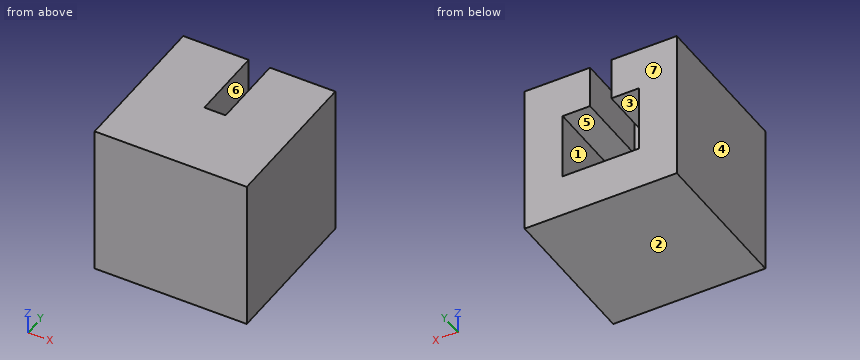
```python
from build123d import *

# Parameters (mm, degrees)
SKETCH1_W           = 12.7
SKETCH1_H           = 12.7
BOSS_EXTRUDE1_DEPTH = 12.7
SKETCH2_W           = 1.778
SKETCH2_H           = 3.560002412
CUT_EXTRUDE1_DEPTH  = 6.35


with BuildPart() as part:
    # Sketch1 → Boss-Extrude1 (new body)
    with BuildSketch(Plane(origin=(0, 0, 0), x_dir=(1, 0, 0), z_dir=(0, 1, 0))):
        Rectangle(SKETCH1_W, SKETCH1_H)
    extrude(amount=BOSS_EXTRUDE1_DEPTH)

    # Sketch2 → Cut-Extrude1 (cut)
    with BuildSketch(Plane(origin=(0, 12.7, 0), x_dir=(1, 0, 0), z_dir=(0, 1, 0))):
        Polygon((-3.175, -2.789997588), (-0.889, -2.789997588), (0.889, -2.789997588), (3.175, -2.789997588), (3.175, 2.789997588), (-3.175, 2.789997588), align=None)
        with Locations((0, -4.569998794)):
            Rectangle(SKETCH2_W, SKETCH2_H)
    extrude(amount=-CUT_EXTRUDE1_DEPTH, mode=Mode.SUBTRACT)


solid = part.part
```
For this review, take the finished solid that the model builds, in its own axes (mm). Face numbers are marked on the shaded views. A direction names the side the tool comes from. Coordinates: 2 decimals unless noted, no trailing zeros. Loops run counter-clockwise (first coordinate to the right, second up) from the corner with the lowest first, then second, coordinate; pieces in that order, holes last. Notation, with made-up numbers: (48.25, 15) - (60.25, 15) arc R22 ccw to (60.25, 40) - close; hole circle Ø3 at (13.25, 21). An arc over 180 degrees is marked (long way). Use one line per item in the form item = value. Start each with the question number.
1) Take a section at B-B (z = 3.5). State the section outline as (x, y) points, plus the area to 3 significant figures.
2) Take a section at A-A (y = 8.25). State the section outline as (x, z) points (3 decimals), plus the area to 3 significant figures.
3) Draft analysis for pull direction Z (two halves, no side actions). For the marked faces 1, 2, 3 and 4, state which applies: released by +Z, released by -Z, zero draft, split by the parting line, or undercut.
4) Take a section at D-D (z = -2). State the section outline as (x, y) points (3 decimals).
5) For the marked faces 5, 6 and 7, list the 3-axis set-ups (+Z, -Z, +X, -X, +Y, -Y) from which the entire face can be reached by the end or side of a thin tool; tool diameter is ignored.
6) Take a section at C-C (x = -0.25). State the section outline as (y, z) points.
7) To check wall thickness, follow probe 1 along X at (y, z) = (7.5, -1.5) (3 decimals); probe 2 along Z at (x, y) = (-3, 11.25); probe 3 along Z at (x, y) = (-0.5, 9.75). State the ranges of each line that lie inside material, in increasing order. Write a range as from..to.
From the geometry:
q1.outline = (-6.35, 0) - (6.35, 0) - (6.35, 12.7) - (0.89, 12.7) - (0.89, 6.35) - (-0.89, 6.35) - (-0.89, 12.7) - (-6.35, 12.7) - close
q1.area = 150 mm2
q2.outline = (-6.35, -6.35) - (6.35, -6.35) - (6.35, 6.35) - (0.889, 6.35) - (0.889, 2.79) - (3.175, 2.79) - (3.175, -2.79) - (-3.175, -2.79) - (-3.175, 2.79) - (-0.889, 2.79) - (-0.889, 6.35) - (-6.35, 6.35) - close
q2.area = 120 mm2
q3.face_1 = undercut
q3.face_2 = released by -Z
q3.face_3 = undercut
q3.face_4 = zero draft
q4.outline = (-6.35, 0) - (6.35, 0) - (6.35, 12.7) - (3.175, 12.7) - (3.175, 6.35) - (-3.175, 6.35) - (-3.175, 12.7) - (-6.35, 12.7) - close
q5.face_5 = +Y
q5.face_6 = +Z, +Y
q5.face_7 = +Z, -Z, +X, -X, +Y
q6.outline = (0, -6.35) - (12.7, -6.35) - (12.7, -2.79) - (6.35, -2.79) - (6.35, 6.35) - (0, 6.35) - close
q7.probe_1 = -6.35..-3.175, 3.175..6.35
q7.probe_2 = -6.35..-2.79, 2.79..6.35
q7.probe_3 = -6.35..-2.79
